from build123d import *

# Parameters (mm, degrees)
F0_W     = 1
F0_H     = 30
F0_W_2   = 38
F0_H_2   = 1.332180649
F1_DEPTH = 140
F2_W     = 40
F2_H     = 0.123128891
F3_DEPTH = 40
F4_W     = 30
F4_H     = 34
F5_DEPTH = 140.123128891


with BuildPart() as f1:
    # F0 (on Front) → F1 (new body)
    with BuildSketch(Plane.XZ):
        Polygon((-19.5, 15), (-20, 15), (-20, -11.8550653383), (-20, -15), (-19.5, -15), (-19.5, -5.2632528394), (-19.5, -3.2632528394), (-19.5, 2.7367471606), (-19.5, 4.7367471606), align=None)
        Polygon((-19, -15), (-19, 15), (-19.5, 15), (-19.5, 4.7367471606), (-19.5, 2.7367471606), (-19.5, -3.2632528394), (-19.5, -5.2632528394), (-19.5, -15), align=None)
        Polygon((-17.5, -17.5), (-20, -15), (-20, -20), (-15, -20), align=None)
        Polygon((-15, -15), (-19, -15), (-19.5, -15), (-20, -15), (-17.5, -17.5), (-16.767766953, -16.767766953), align=None)
        Polygon((-15, -17.5), (-15, -15), (-16.767766953, -16.767766953), (-17.5, -17.5), (-15, -20), align=None)
        with BuildLine():
            Line((15, -15), (-15, -15))
            Line((-15, -15), (-15, -17.5))
            Line((-15, -17.5), (-11.391207267, -17.5))
            ThreePointArc((-11.391207267, -17.5), (-10.2485464886, -16.3573392216), (-9.1058857102, -17.5))
            Line((-9.1058857102, -17.5), (-7.9234171988, -17.5))
            ThreePointArc((-7.9234171988, -17.5), (-5.948765669, -15.5253484702), (-3.9741141393, -17.5))
            Line((-3.9741141393, -17.5), (3.9741141393, -17.5))
            ThreePointArc((3.9741141393, -17.5), (5.948765669, -15.5253484702), (7.9234171988, -17.5))
            Line((7.9234171988, -17.5), (9.1058857102, -17.5))
            ThreePointArc((9.1058857102, -17.5), (10.2485464886, -16.3573392216), (11.391207267, -17.5))
            Line((11.391207267, -17.5), (15, -17.5))
            Line((15, -17.5), (15, -15))
        make_face()
        with BuildLine():
            Line((-15, -20), (15, -20))
            Line((15, -20), (15, -17.5))
            Line((15, -17.5), (11.391207267, -17.5))
            ThreePointArc((11.391207267, -17.5), (10.2485464886, -18.6426607784), (9.1058857102, -17.5))
            Line((9.1058857102, -17.5), (7.9234171988, -17.5))
            ThreePointArc((7.9234171988, -17.5), (5.948765669, -19.4746515298), (3.9741141393, -17.5))
            Line((3.9741141393, -17.5), (-3.9741141393, -17.5))
            ThreePointArc((-3.9741141393, -17.5), (-5.948765669, -19.4746515298), (-7.9234171988, -17.5))
            Line((-7.9234171988, -17.5), (-9.1058857102, -17.5))
            ThreePointArc((-9.1058857102, -17.5), (-10.2485464886, -18.6426607784), (-11.391207267, -17.5))
            Line((-11.391207267, -17.5), (-15, -17.5))
            Line((-15, -17.5), (-15, -20))
        make_face()
        with BuildLine():
            Line((-9.1058857102, -17.5), (-11.391207267, -17.5))
            ThreePointArc((-11.391207267, -17.5), (-10.2485464886, -18.6426607784), (-9.1058857102, -17.5))
        make_face()
        with BuildLine():
            ThreePointArc((-9.1058857102, -17.5), (-10.2485464886, -16.3573392216), (-11.391207267, -17.5))
            Line((-11.391207267, -17.5), (-9.1058857102, -17.5))
        make_face()
        with BuildLine():
            ThreePointArc((-3.9741141393, -17.5), (-5.948765669, -15.5253484702), (-7.9234171988, -17.5))
            Line((-7.9234171988, -17.5), (-3.9741141393, -17.5))
        make_face()
        with BuildLine():
            Line((-3.9741141393, -17.5), (-7.9234171988, -17.5))
            ThreePointArc((-7.9234171988, -17.5), (-5.948765669, -19.4746515298), (-3.9741141393, -17.5))
        make_face()
        with BuildLine():
            Line((3.9741141393, -17.5), (7.9234171988, -17.5))
            ThreePointArc((7.9234171988, -17.5), (5.948765669, -15.5253484702), (3.9741141393, -17.5))
        make_face()
        with BuildLine():
            ThreePointArc((3.9741141393, -17.5), (5.948765669, -19.4746515298), (7.9234171988, -17.5))
            Line((7.9234171988, -17.5), (3.9741141393, -17.5))
        make_face()
        Polygon((19, 17.5), (-19, 17.5), (-19, 15), (-19, -15), (-15, -15), (15, -15), (19, -15), (19, 15), align=None)
        with BuildLine():
            ThreePointArc((9.1058857102, -17.5), (10.2485464886, -18.6426607784), (11.391207267, -17.5))
            Line((11.391207267, -17.5), (9.1058857102, -17.5))
        make_face()
        with BuildLine():
            Line((9.1058857102, -17.5), (11.391207267, -17.5))
            ThreePointArc((11.391207267, -17.5), (10.2485464886, -16.3573392216), (9.1058857102, -17.5))
        make_face()
        Polygon((20, -20), (20, -15), (19, -15), (15, -15), (15, -17.5), (15, -20), align=None)
        with Locations((19.5, 0)):
            Rectangle(F0_W, F0_H)
        Polygon((-19, 18.832180649), (-19, 20), (-20, 20), (-20, 15), (-19.5, 15), (-19, 15), (-19, 17.5), align=None)
        with Locations((0, 18.1660903245)):
            Rectangle(F0_W_2, F0_H_2)
        Polygon((15, 20), (-15, 20), (-19, 20), (-19, 18.832180649), (19, 18.832180649), (19, 20), align=None)
        Polygon((20, 20), (19, 20), (19, 18.832180649), (19, 17.5), (19, 15), (20, 15), align=None)
    extrude(amount=F1_DEPTH)

    # F2 (on face) → F3 (join, through all)
    with BuildSketch(Plane.XY.offset(20)):
        with Locations((0, -140.0615644455)):
            Rectangle(F2_W, F2_H)
        Polygon((-20, -140.123128891), (-20, -140), (-20, 0), (-30, -140.123128891), align=None)
        Polygon((20, 0), (20, -140), (20, -140.123128891), (30, -140.123128891), align=None)
    extrude(amount=-F3_DEPTH)

    # F4 (on face) → F5 (cut, through all)
    with BuildSketch(Plane(origin=(0, 0, 0), x_dir=(-1, 0, 0), z_dir=(0, 1, 0))):
        Rectangle(F4_W, F4_H)
    extrude(amount=-F5_DEPTH, mode=Mode.SUBTRACT)


solid = f1.part
Design review of the part built by this model. Coordinates are the model's own, in mm. A direction names the side the tool comes from. Give positions to 0.01 mm unless a question says otherwise; leave off trailing zeros. Loops run counter-clockwise (first coordinate to the right, second up) from the corner with the lowest first, then second, coordinate; pieces in that order, holes last. Notation, with made-up numbers: M 6.5,42.5 L 39.5,42.5 A25 ccw 39.5,67.5 Z; hole C 76,-1 d2. An arc over 180 degrees is marked long. Write item = value, one per line.
Q1. To check wall thickness, follow line 1 (Z direction, x = 4.5, y = -121); line 2 (X direction, y = -9, z = -6); line 3 (X direction, y = -14, z = 1). State the ranges of each line that lie inside material, in increasing order. Write a range as [from, to].
Output values:
line_1 = [-20, -17], [17, 20]
line_2 = [-20.64, -15], [15, 20.64]
line_3 = [-21, -15], [15, 21]
Q2. For faces 1 (the flat face through (-24.93, -69.08, 0.28)), 2 (the flat face through (-15, -69, 0)), list the 3-axis set-ups (+Z, -Z, +X, -X, +Y, -Y) from which the entire face can be reached by the end or side of a thin tool; tool diameter is ignored.
Output values:
face_1 = +Z, -Z, -X, +Y
face_2 = +Y, -Y
Q3. Draft analysis for pull direction Z (two halves, no side actions). For faces 3 (the flat face through (25.07, -71.04, 0.28)), 4 (the flat face through (0, -69, -20)), 5 (the flat face through (15, -69, 0)), 6 (the flat face through (0, -69, 20)), state which applies: +Z half, -Z half, draft (parallel to the pull), parting line (faces both ways), or undercut.
Output values:
face_3 = draft
face_4 = -Z half
face_5 = undercut
face_6 = +Z half
Q4. We need section D-D (y = -18.5). Give the boundary of the cut face in (x, z).
Output values:
outline = M -21.32,-20 L 21.32,-20 L 21.32,20 L -21.32,20 Z; hole M -15,-17 L 15,-17 L 15,17 L -15,17 Z
Q5. We need section C-C (y = -59.5). Give the boundary of the cut face in (x, z), plus the area to 3 significant figures.
Output values:
outline = M -24.25,-20 L 24.25,-20 L 24.25,20 L -24.25,20 Z; hole M -15,-17 L 15,-17 L 15,17 L -15,17 Z
area = 920 mm^2
Q6. We need section A-A (x = -2). Give the boundary of the cut face in (y, z).
Output values:
outline = M -140.12,-20 L 0,-20 L 0,-17 L -140.12,-17 Z; M -140.12,17 L 0,17 L 0,20 L -140.12,20 Z
Q7. Insertion check: pin 1 (1.5 mm diameter, centred on y = -109, z = 8.5, fed in from +X); pin 2 (17 mm diameter, centred on y = -50, z = -5.5, fed in from +X); pin 3 (10 mm diameter, centred on y = -62.5, z = -2.5, fed in from -X). Each pin has a flat end and moves straight along its axis. Give the tip position at first contact, or say it passes through.
Output values:
pin_1 = 27.83
pin_2 = 24.17
pin_3 = -24.82
Q8. We need section B-B (z = 9.5). Give the boundary of the cut face in (x, y).
Output values:
outline = M -30,-140.12 L -15,-140.12 L -15,0 L -20,0 Z; M 15,-140.12 L 30,-140.12 L 20,0 L 15,0 Z
